from build123d import *

# Parameters (mm, degrees)
SKETCH_1_W          = 105
SKETCH_1_H          = 80
EXTRUDE_1_DEPTH     = 5
SKETCH_2_R          = 1.5
CUT_EXTRUDE_1_DEPTH = 67.191011474
SKETCH_3_R          = 2
CUT_EXTRUDE_2_DEPTH = 5
FILLET_1_R          = 10


with BuildPart() as part:
    # 草图1 → 凸台-拉伸1 (new body)
    with BuildSketch(Plane(origin=(0, 0, 0), x_dir=(1, 0, 0), z_dir=(0, 1, 0))):
        Rectangle(SKETCH_1_W, SKETCH_1_H)
    extrude(amount=EXTRUDE_1_DEPTH)

    # 草图2 → 切除-拉伸1 (cut, through all)
    with BuildSketch(Plane(origin=(0, 5, 0), x_dir=(1, 0, 0), z_dir=(0, 1, 0))):
        with Locations(Location((-17.5, 20, 0), (0, 0, 270))):
            Circle(SKETCH_2_R)
        with Locations(Location((27.5, 20, 0), (0, 0, 270))):
            Circle(SKETCH_2_R)
        with Locations(Location((27.5, -2, 0), (0, 0, 270))):
            Circle(SKETCH_2_R)
        with Locations(Location((-17.5, -2, 0), (0, 0, 270))):
            Circle(SKETCH_2_R)
    extrude(amount=-CUT_EXTRUDE_1_DEPTH, mode=Mode.SUBTRACT)

    # 草图3 → 切除-拉伸2 (cut)
    with BuildSketch(Plane(origin=(0, 5, 0), x_dir=(1, 0, 0), z_dir=(0, 1, 0))):
        with Locations(Location((-12.5, -30, 0), (0, 0, 270))):
            Circle(SKETCH_3_R)
        with Locations(Location((-42.5, -30, 0), (0, 0, 270))):
            Circle(SKETCH_3_R)
        with Locations(Location((42.5, 0, 0), (0, 0, 270))):
            Circle(SKETCH_3_R)
        with Locations(Location((42.5, 30, 0), (0, 0, 270))):
            Circle(SKETCH_3_R)
        with Locations(Location((42.5, -30, 0), (0, 0, 270))):
            Circle(SKETCH_3_R)
    extrude(amount=-CUT_EXTRUDE_2_DEPTH, mode=Mode.SUBTRACT)

    # 圆角1
    fillet_1_edges = [part.edges().sort_by_distance(p)[0] for p in [
        (-52.5, 2.5, -40),
        (52.5, 2.5, -40),
        (52.5, 2.5, 40),
        (-52.5, 2.5, 40),
    ]]
    fillet(fillet_1_edges, radius=FILLET_1_R)


solid = part.part
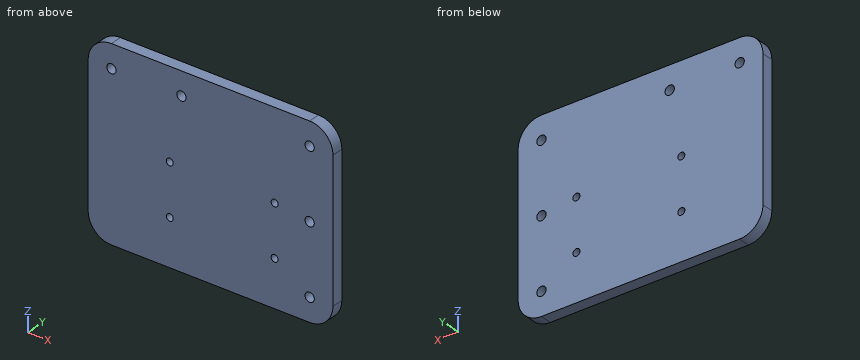
Work out the finished part from the listing and answer in its coordinate system (mm). Give positions to 0.01 mm unless a question says otherwise; leave off trailing zeros. Loops run counter-clockwise (first coordinate to the right, second up) from the corner with the lowest first, then second, coordinate; pieces in that order, holes last. Notation, with made-up numbers: (-26.75, 2) -> (-4.75, 2) arc R25 ccw to (-4.75, 40) -> close; hole circle Ø7 at (61, 44). An arc over 180 degrees is marked (long way). Use a Markdown table: item, result. Add a question column.
1) The part is cut by section D-D, the plane z = 34.5. Determine the outline of the cut face in (x, y), plus the area to 3 significant figures.
2) The part is cut by section C-C, the plane x = 27.5. Determine the outline of the cut face in (y, z), plus the area to 3 significant figures.
3) Consider line 1 along X through (y, z) = (3.2, -20); line 2 along Z through (x, y) = (28, 2.4); line 3 along Z through (x, y) = (44, 0.4). Determine where each line is inside the solid, lowest interval first.
4) The part is cut by section A-A, the plane z = -20. Determine the outline of the cut face in (x, y).
5) The part is cut by section B-B, the plane y = 3.25. Count the separate pieces of the cut face and the enclosed holes in it, plus the area to 3 significant figures.
Reported:
| question | item | result |
|---|---|---|
| 1 | outline | (-51.43, 0) -> (51.43, 0) -> (51.43, 5) -> (-51.43, 5) -> close |
| 1 | area | 514 mm^2 |
| 2 | outline | (0, -40) -> (5, -40) -> (5, -21.5) -> (0, -21.5) -> close; (0, -18.5) -> (5, -18.5) -> (5, 0.5) -> (0, 0.5) -> close; (0, 3.5) -> (5, 3.5) -> (5, 40) -> (0, 40) -> close |
| 2 | area | 370 mm^2 |
| 3 | line 1 | x = -52.5 to -19, -16 to 26, 29 to 52.5 |
| 3 | line 2 | z = -40 to -21.41, -18.59 to 0.59, 3.41 to 40 |
| 3 | line 3 | z = -39.89 to -31.32, -28.68 to -1.32, 1.32 to 28.68, 31.32 to 39.89 |
| 4 | outline | (-52.5, 0) -> (-19, 0) -> (-19, 5) -> (-52.5, 5) -> close; (-16, 0) -> (26, 0) -> (26, 5) -> (-16, 5) -> close; (29, 0) -> (52.5, 0) -> (52.5, 5) -> (29, 5) -> close |
| 5 | separate pieces | 1 |
| 5 | enclosed holes | 9 |
| 5 | area | 8,220 mm^2 |
